Source: CAD feature listing. Evaluate the final solid. Frame: model axes, mm. A direction names the side the tool comes from. Give positions to 0.01 mm unless a question says otherwise; leave off trailing zeros. Write each loop counter-clockwise with the first axis right and the second up, starting at its lowest first coordinate (ties: lowest second). Pieces come first, ordered by that corner, then holes. Notation, with made-up numbers: (-34.5, 88) -> (7.5, 88) arc R19 cw to (7.5, 125) -> close; hole circle Ø4 at (73.5, 87.25). An arc over 180 degrees is marked (long way). Write item = value, one per line.
from build123d import *

# Parameters (mm, degrees)
F0_R     = 12.5
F1_DEPTH = 30
F2_R     = 12.5
F3_DEPTH = 27.5
F4_R     = 10
F5_DEPTH = 30
F6_R     = 10
F7_DEPTH = 45


with BuildPart() as f1:
    # F0 (on Right) → F1 (new body, symmetric)
    with BuildSketch(Plane.YZ):
        Circle(F0_R)
    extrude(amount=F1_DEPTH, both=True)

    # F2 (on Top) → F3 (join)
    with BuildSketch(Plane.XY):
        Circle(F2_R)
    extrude(amount=F3_DEPTH)

    # F4 (on Right) → F5 (cut, symmetric)
    with BuildSketch(Plane.YZ):
        Circle(F4_R)
    extrude(amount=F5_DEPTH, both=True, mode=Mode.SUBTRACT)

    # F6 (on Top) → F7 (cut)
    with BuildSketch(Plane.XY):
        Circle(F6_R)
    extrude(amount=F7_DEPTH, mode=Mode.SUBTRACT)


solid = f1.part
(1) Section query D-D (z = 15). Return loops of the section in (x, y), plus the area to 3 significant figures.
Values follow:
outline = circle Ø25 at (0, 0); hole circle Ø20 at (0, 0)
area = 177 mm2
(2) Section query A-A (y = 0). Return loops of the section in (x, z).
Values follow:
outline = (-30, -12.5) -> (30, -12.5) -> (30, -10) -> (-30, -10) -> close; (-30, 10) -> (-10, 10) -> (-10, 27.5) -> (-12.5, 27.5) -> (-12.5, 12.5) -> (-30, 12.5) -> close; (10, 10) -> (30, 10) -> (30, 12.5) -> (12.5, 12.5) -> (12.5, 27.5) -> (10, 27.5) -> close
(3) Section query C-C (x = 0). Return loops of the section in (y, z).
Values follow:
outline = (-12.5, 0) arc R12.5 ccw to (12.5, 0) -> (12.5, 27.5) -> (10, 27.5) -> (10, 0) arc R10 cw to (-10, 0) -> (-10, 27.5) -> (-12.5, 27.5) -> close
(4) Pull-direction query (Y, two-part tool) for faces 3 (the face through (0.42, 5.77, -11.09)), 4 (the face through (-0.1, 10.2, 27.5)), 5 (the face through (0.42, -2.17, -9.76)); classes: pulls with the +Y half, pulls with the -Y half, needs draft (parallel to the pull), parting line crosses it, or undercut.
Values follow:
face_3 = parting line crosses it
face_4 = needs draft
face_5 = undercut
(5) Access query for faces 1 (the face through (30, -0.1, 10.2)), 2 (the face through (-12.488, 0.55, 16.613)). Directions: +Z, -Z, +X, -X, +Y, -Y. A direction counts if a zero-diameter tool reaches every point of the face in a straight line with its end or side. Return the directions, or none.
Values follow:
face_1 = +Z, -Z, +X, +Y, -Y
face_2 = +Z
(6) Material intervals for line 1 (X direction, y = 0, z = 14.5), sorted ascending.
Values follow:
line_1 = -12.5 to -10, 10 to 12.5
(7) Section query B-B (z = 6). Return loops of the section in (x, y), plus the area to 3 significant figures.
Values follow:
outline = (-30, -10.97) -> (-6, -10.97) arc R12.5 ccw to (6, -10.97) -> (30, -10.97) -> (30, -8) -> (6, -8) arc R10 cw to (-6, -8) -> (-30, -8) -> close; (-30, 8) -> (-6, 8) arc R10 cw to (6, 8) -> (30, 8) -> (30, 10.97) -> (6, 10.97) arc R12.5 ccw to (-6, 10.97) -> (-30, 10.97) -> close
area = 348 mm2
(8) First-contact query: pin 1 (10 mm diameter, centred on x = -15, y = -0.5, fed in from +Z); pin 2 (4 mm diameter, centred on x = -16, z = 16, fed in from -Y); pin 3 (4 mm diameter, centred on y = -8, z = 15.5, fed in from +X); pin 4 (2 mm diameter, centred on x = -5.5, y = 2.5, fed in from +Z). Flat tips, straight axial feed; report the tip coordinate or a pass-through.
Values follow:
pin_1 = 27.5
pin_2 = through
pin_3 = 10.97
pin_4 = -9.37
